from build123d import *

# Parameters (mm, degrees)
F1_DEPTH = 63.5
F2_DEPTH = 25.4
F3_DEPTH = 7.9375


with BuildPart() as f1:
    # F0 (on Front) → F1 (new body, symmetric)
    with BuildSketch(Plane.XZ):
        Polygon((-41.275, -9.525), (41.275, -9.525), (41.275, 9.525), (22.225, 9.525), (-41.275, 9.525), align=None)
    extrude(amount=F1_DEPTH, both=True)

    # F0 (on Front) → F2 (join, symmetric)
    with BuildSketch(Plane.XZ):
        with BuildLine():
            Line((22.225, 9.525), (41.275, 9.525))
            Line((41.275, 9.525), (41.275, 27.2855908291))
            ThreePointArc((41.275, 27.2855908291), (44.9109862911, 37.3960887611), (54.1533834246, 42.8752))
            Line((54.1533834246, 42.8752), (60.325, 42.8752))
            Line((60.325, 42.8752), (60.325, 61.9252))
            Line((60.325, 61.9252), (52.6943180668, 61.9252))
            ThreePointArc((52.6943180668, 61.9252), (30.926248204, 50.3522435282), (22.225, 27.2855908291))
            Line((22.225, 27.2855908291), (22.225, 9.525))
        make_face()
    extrude(amount=F2_DEPTH, both=True)

    # F0 (on Front) → F3 (join, symmetric)
    with BuildSketch(Plane.XZ):
        with BuildLine():
            add(Edge.make_bspline(
                [(52.6943180668, 61.9252), (15.7995279878, 57.229410857), (-21.768245846, 41.0787798464), (-41.275, 9.525)],
                knots=[0, 0, 0, 0, 107.5918849076, 107.5918849076, 107.5918849076, 107.5918849076], degree=3))
            Line((-41.275, 9.525), (22.225, 9.525))
            Line((22.225, 9.525), (22.225, 27.2855908291))
            ThreePointArc((22.225, 27.2855908291), (30.926248204, 50.3522435282), (52.6943180668, 61.9252))
        make_face()
    extrude(amount=F3_DEPTH, both=True)


solid = f1.part
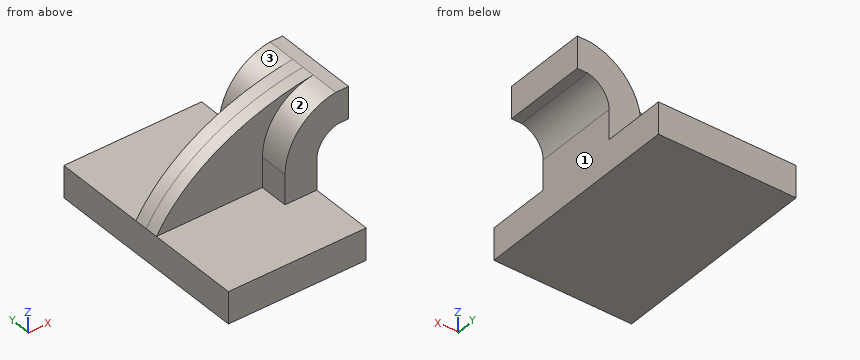
For this review, take the finished solid that the model builds, in its own axes (mm). Face numbers are marked on the shaded views. A direction names the side the tool comes from. Round coordinates to 2 decimals unless told otherwise and drop trailing zeros. Write each loop counter-clockwise with the first axis right and the second up, starting at its lowest first coordinate (ties: lowest second). Pieces come first, ordered by that corner, then holes. Notation, with made-up numbers: (10.5, -38.75) - (46.5, -38.75) arc R28 ccw to (46.5, -9.75) - close; hole circle Ø11 at (16, -4.5). An arc over 180 degrees is marked (long way). Write item = value, one per line. Start each with the question number.
1. Consider section B-B on z = 7.5. State the section outline as (x, y) points (3 decimals).
2. For the marked faces 1, 2 and 3, list the 3-axis set-ups (+Z, -Z, +X, -X, +Y, -Y) from which the entire face can be reached by the end or side of a thin tool; tool diameter is ignored.
3. For pin 1 Ø5 at (y, z) = (-16, 18) entering from -X (3 decimals); pin 2 Ø5 at (x, y) = (0, -24) entering from +Z (3 decimals); pin 3 Ø2 at (y, z) = (-3.5, 2) entering from +X (3 decimals), all flat-tipped, find the tip position at first contact; note any pin that passes through.
4. Wall thickness on L1, parallel to Y at x = -5, z = 10.5; L2, parallel to Z at x = -15, y = 52.5 (3 decimals); L3, parallel to X at y = 15, z = -5 (3 decimals): over which ranges is each line inside the solid? List them lowest first.
5. Consider section A-A on y = -20. State the section outline as (x, z) points (3 decimals).
6. Consider section C-C on y = -37.5. State the section outline as (x, z) points (3 decimals), plus the area to 3 significant figures.
Evaluation:
q1.outline = (-41.275, -63.5) - (41.275, -63.5) - (41.275, 63.5) - (-41.275, 63.5) - close
q2.face_1 = -Z, +X, +Y, -Y
q2.face_2 = +Z, -X, -Y
q2.face_3 = +Z, -X, +Y
q3.pin_1 = 22.225
q3.pin_2 = 9.525
q3.pin_3 = 41.275
q4.L1 = -7.94 to 7.94
q4.L2 = -9.525 to 9.525
q4.L3 = -41.275 to 41.275
q5.outline = (-41.275, -9.525) - (41.275, -9.525) - (41.275, 27.286) arc R15.875 cw to (54.153, 42.875) - (60.325, 42.875) - (60.325, 61.925) - (52.694, 61.925) arc R34.925 ccw to (22.225, 27.286) - (22.225, 9.525) - (-41.275, 9.525) - close
q6.outline = (-41.275, -9.525) - (41.275, -9.525) - (41.275, 9.525) - (-41.275, 9.525) - close
q6.area = 1,570 mm2
